CAD build for the part. Positions are in the model's coordinates, mm. Coordinates: 2 decimals unless noted, no trailing zeros. Write each loop counter-clockwise with the first axis right and the second up, starting at its lowest first coordinate (ties: lowest second). Pieces come first, ordered by that corner, then holes. Notation, with made-up numbers: (27, 16) - (81, 16) arc R26 ccw to (81, 54) - close; hole circle Ø4 at (66, 74). An arc over 180 degrees is marked (long way). Answer in a Markdown table with one row per item. Add a question column.
Q1. Drill centre lines: line 1 along Y through (x, z) = (13, 0.2); line 2 along X through (y, z) = (211.15, 0.3); line 3 along X through (y, z) = (189, 0.4). Where is each one in solid material? Low to high. Write a range as from..to.
Q2. Pin check, flat tips, straight feed: pin 1 (0.5 mm diameter, centred on x = 149.5, z = 0.5, fed in from +Y); pin 2 (6 mm diameter, centred on x = 13, y = 10.85, fed in from -Z). Stop position of each tip, or through.
Q3. Band-saw the part on B-B (z = 0.7). State how many separate pieces and enclosed holes the cut face has, and give its area (3 significant figures).
Q4. Band-saw the part on C-C (y = 49). List the corners of the cut face in (x, z).
Q5. Band-saw the part on D-D (x = 247). List the corners of the cut face in (y, z), and give its area (3 significant figures).
Q6. Band-saw the part on A-A (y = 182). List the corners of the cut face in (x, z), and give its area (3 significant figures).
```python
from build123d import *

# Parameters (mm, degrees)
SKETCH1_R                     = 2.5
SKETCH1_W                     = 7
SKETCH1_H                     = 5
F_1MM_STAINLESS_STEAL_DEPTH   = 1
SKETCH3_R                     = 1.25
CUT_EXTRUDE2_DEPTH            = 356.648703077
FILLET2_1MM_STAINLESS_STEAL_R = 0.5


with BuildPart() as part:
    # Sketch1 → 1mm Stainless_Steal (new body)
    with BuildSketch(Plane.XY):
        with BuildLine():
            Line((77, 218), (77, 55))
            ThreePointArc((77, 55), (79.928932188, 47.928932188), (87, 45))
            Line((87, 45), (243, 45))
            ThreePointArc((243, 45), (250.071067812, 47.928932188), (253, 55))
            Line((253, 55), (253, 218))
            Line((253, 218), (281, 218))
            Line((281, 218), (281, 0))
            Line((281, 0), (0, 0))
            Line((0, 0), (0, 218))
            Line((0, 218), (77, 218))
        make_face()
        with Locations((13, 10.85)):
            Circle(SKETCH1_R, mode=Mode.SUBTRACT)
        with Locations((13, 211.15)):
            Circle(SKETCH1_R, mode=Mode.SUBTRACT)
        with Locations((56, 189)):
            Circle(SKETCH1_R, mode=Mode.SUBTRACT)
        with Locations((268, 10.85)):
            Circle(SKETCH1_R, mode=Mode.SUBTRACT)
        with Locations((273, 189)):
            Circle(SKETCH1_R, mode=Mode.SUBTRACT)
        with Locations((64.5, 12.5)):
            Rectangle(SKETCH1_W, SKETCH1_H, mode=Mode.SUBTRACT)
    extrude(amount=F_1MM_STAINLESS_STEAL_DEPTH)

    # Sketch3 → Cut-Extrude2 (cut, through all)
    with BuildSketch(Plane.XY.offset(1)):
        with Locations((61.883883476, 14.116116524)):
            Circle(SKETCH3_R)
        with Locations((67.116116524, 10.883883476)):
            Circle(SKETCH3_R)
        with Locations((67.116116524, 14.116116524)):
            Circle(SKETCH3_R)
        with Locations((61.883883476, 10.883883476)):
            Circle(SKETCH3_R)
    extrude(amount=-CUT_EXTRUDE2_DEPTH, mode=Mode.SUBTRACT)

    # Fillet2_1mm_Stainless_Steal
    fillet2_1mm_stainless_steal_edges = [part.edges().sort_by_distance(p)[0] for p in [
        (253, 218, 0.5),
        (281, 218, 0.5),
        (281, 0, 0.5),
        (0, 0, 0.5),
        (0, 218, 0.5),
        (77, 218, 0.5),
    ]]
    fillet(fillet2_1mm_stainless_steal_edges, radius=FILLET2_1MM_STAINLESS_STEAL_R)


solid = part.part
```
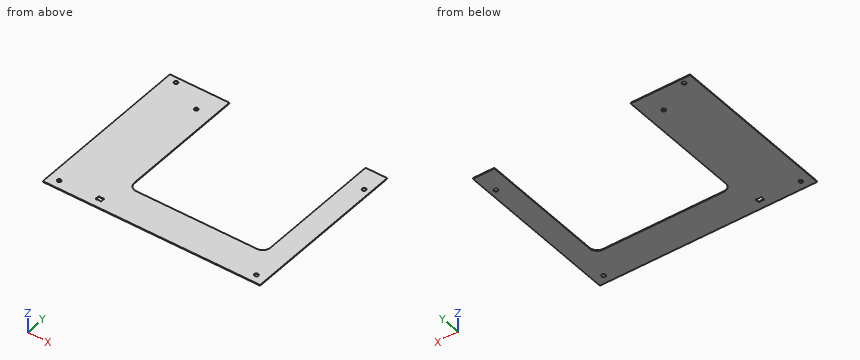
Checked values:
| question | item | result |
|---|---|---|
| 1 | line 1 | y = 0..8.35, 13.35..208.65, 213.65..218 |
| 1 | line 2 | x = 0..10.5, 15.5..77, 253..281 |
| 1 | line 3 | x = 0..53.5, 58.5..77, 253..270.5, 275.5..281 |
| 2 | pin 1 | stops at y = 45 |
| 2 | pin 2 | stops at z = 0 |
| 3 | separate pieces | 1 |
| 3 | enclosed holes | 6 |
| 3 | area | 30,700 mm² |
| 4 | outline | (0, 0) - (79, 0) - (79, 1) - (0, 1) - close; (251, 0) - (281, 0) - (281, 1) - (251, 1) - close |
| 5 | outline | (0, 0) - (45.83, 0) - (45.83, 1) - (0, 1) - close |
| 5 | area | 45.8 mm² |
| 6 | outline | (0, 0) - (77, 0) - (77, 1) - (0, 1) - close; (253, 0) - (281, 0) - (281, 1) - (253, 1) - close |
| 6 | area | 105 mm² |
